Verification items for the finished model (mm, model axes). Face numbers are marked on the shaded views. A direction names the side the tool comes from. Give positions to 0.01 mm unless a question says otherwise; leave off trailing zeros. Write each loop counter-clockwise with the first axis right and the second up, starting at its lowest first coordinate (ties: lowest second). Pieces come first, ordered by that corner, then holes.
Autodesk Inventor part; units mm, degrees
ref_plane "YZ Plane" through (0, 0, 0) normal (1, 0, 0) x (0, 1, 0)
ref_plane "XZ Plane" through (0, 0, 0) normal (0, 1, 0) x (-1, 0, 0)
ref_plane "XY Plane" through (0, 0, 0) normal (0, 0, 1) x (1, 0, 0)
sketch "Sketch1" plane through (0, 0, 0) normal (0, 1, 0) x (-1, 0, 0)
  line L0 (-19.05, -74.6125) -> (19.05, -74.6125)
  line L1 (19.05, -74.6125) -> (19.05, 74.6125)
  line L2 (19.05, 74.6125) -> (-19.05, 74.6125)
  line L3 (-19.05, 74.6125) -> (-19.05, -74.6125)
  line L4 (-19.05, -74.6125) -> (19.05, 74.6125) construction
  line L5 (19.05, -74.6125) -> (-19.05, 74.6125) construction
  circle A0 centre (0, 66.675) radius 2.75
  circle A1 centre (0, -66.675) radius 2.75
  line L6 (-12.7, -50.8) -> (12.7, -50.8)
  line L7 (12.7, -50.8) -> (12.7, 50.8)
  line L8 (12.7, 50.8) -> (-12.7, 50.8)
  line L9 (-12.7, 50.8) -> (-12.7, -50.8)
  line L10 (-12.7, -50.8) -> (12.7, 50.8) construction
  line L11 (12.7, -50.8) -> (-12.7, 50.8) construction
  circle A2 centre (0, -15.24) radius 3.175
  circle A3 centre (0, -45.72) radius 3.175
  circle A4 centre (0, 15.24) radius 3.175
  circle A5 centre (0, 45.72) radius 3.175
  point P0 (0, 0)
  point P1 (0, 50.8)
  dimension "d0" = 38.1
  dimension "d1" = 149.225
  dimension "d2" = 133.35
  dimension "d3" = 5.5
  dimension "d4" = 5.5
  dimension "d7" = 25.4
  dimension "d8" = 101.6
  dimension "d9" = 6.35
  dimension "d10" = 6.35
  dimension "d11" = 6.35
  dimension "d12" = 6.35
  dimension "d13" = 30.48
  dimension "d14" = 30.48
  dimension "d16" = 5.08
  dimension "d17" = 5.08
  dimension "d19" = 30.48
  dimension "d20" = 66.675
extrude "Extrusion1" add sketch "Sketch1" along normal blind 10.16 contours L3 L2 L1 L0 | L9 L8 L7 L6 | A2 | A3 | A4 | A5
extrude "Extrusion2" add sketch "Sketch1" along normal blind 29.464 contours L9 L8 L7 L6
extrude "Extrusion3" add sketch "Sketch1" along normal blind 48.514 contours A2 | A3 | A4 | A5
sketch "Sketch2" plane through (0, 10.16, 0) normal (0, 1, 0) x (1, 0, 0)
  circle A0 centre (0, -66.675) radius 4.875
  circle A1 centre (0, -66.675) radius 2.75
  circle A2 centre (0, 66.675) radius 4.875
  circle A3 centre (0, 66.675) radius 2.75
  point P0 (0, 0)
  dimension "d25" = 9.75
  dimension "d26" = 9.75
extrude "Extrusion4" cut sketch "Sketch2" against normal blind 5 contours A0 | A2 | A3
fillet "Fillet1" radius 0.3175 8 edges at (12.7, 19.812, 50.8) (-12.7, 19.812, 50.8) (12.7, 19.812, -50.8) (-12.7, 19.812, -50.8) (12.7, 10.16, 0) (0, 10.16, 50.8) (-12.7, 10.16, 0) (0, 10.16, -50.8)
fillet "Fillet2" radius 3.175 4 edges at (19.05, 5.08, 74.6125) (-19.05, 5.08, 74.6125) (19.05, 5.08, -74.6125) (-19.05, 5.08, -74.6125)
fillet "Fillet3" radius 1.27 2 edges at (-4.875, 10.16, 66.675) (-4.875, 10.16, -66.675)
equation "\"d4\" = d3"
equation "\"d10\" = d9"
equation "\"d11\" = d9"
equation "\"d12\" = d9"
properties part number "BlueSea_BusBar"
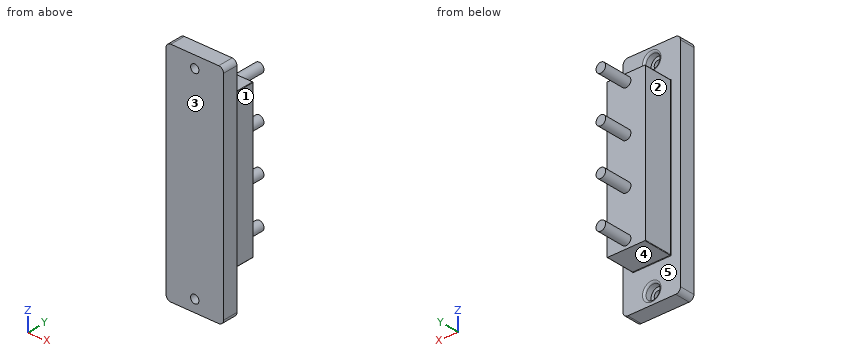
Item 1: Sectioned sample at B-B on y = 43.5. Record the cut outline in (x, z) (3 decimals), then the cut area to 3 significant figures.
Answer key:
outline: circle Ø6.35 at (0, -45.72); circle Ø6.35 at (0, -15.24); circle Ø6.35 at (0, 15.24); circle Ø6.35 at (0, 45.72)
area: 127 mm2
Item 2: Depth check by flat-ended pin: pin 1 (5.5 mm diameter, centred on x = 5.5, y = 20, fed in from +Z); pin 2 (9.5 mm diameter, centred on y = 22, z = -25, fed in from -X); pin 3 (9.5 mm diameter, centred on x = 2.5, y = 17.5, fed in from -Z). Enter the tip coordinate at first touch or a pass-through.
Answer key:
pin 1: stops at z = 50.8
pin 2: stops at x = -12.7
pin 3: stops at z = -50.8
Item 3: Sectioned sample at D-D on y = 19.5. Record the cut outline in (x, z) (1 decimal), then the cut area to 3 significant figures.
Answer key:
outline: (-12.7, -50.5) arc R0.3 ccw to (-12.4, -50.8) - (12.4, -50.8) arc R0.3 ccw to (12.7, -50.5) - (12.7, 50.5) arc R0.3 ccw to (12.4, 50.8) - (-12.4, 50.8) arc R0.3 ccw to (-12.7, 50.5) - close
area: 2,580 mm2
Item 4: Scan lines: line 1 along Z through (x, y) = (0, 8.15); line 2 along Z through (x, y) = (0, 2.75) (1 decimal); line 3 along Z through (x, y) = (4.5, 25). Record each from-to range of solid material in increasing order.
Answer key:
line 1: z = -74.61 to -71.55, -61.8 to 61.8, 71.55 to 74.61
line 2: z = -74.6 to -69.4, -63.9 to 63.9, 69.4 to 74.6
line 3: z = -50.8 to 50.8
Item 5: Set-up check for the marked faces 1, 2, 3, 4 and 5: record each of +Z, -Z, +X, -X, +Y, -Y from which the full face is reachable in a straight line by a thin tool's end or side.
Answer key:
face 1: +Z, -Z, +X, +Y
face 2: +Z, -Z, -X, +Y
face 3: +Z, -Z, +X, -X, -Y
face 4: -Z, +X, -X, +Y
face 5: +Y
Item 6: Sectioned sample at A-A on x = -8.5. Record the cut outline in (y, z) (1 decimal).
Answer key:
outline: (0, -74.6) - (10.2, -74.6) - (10.2, -51.1) arc R0.3 cw to (10.5, -50.8) - (29.5, -50.8) - (29.5, 50.8) - (10.5, 50.8) arc R0.3 cw to (10.2, 51.1) - (10.2, 74.6) - (0, 74.6) - close
